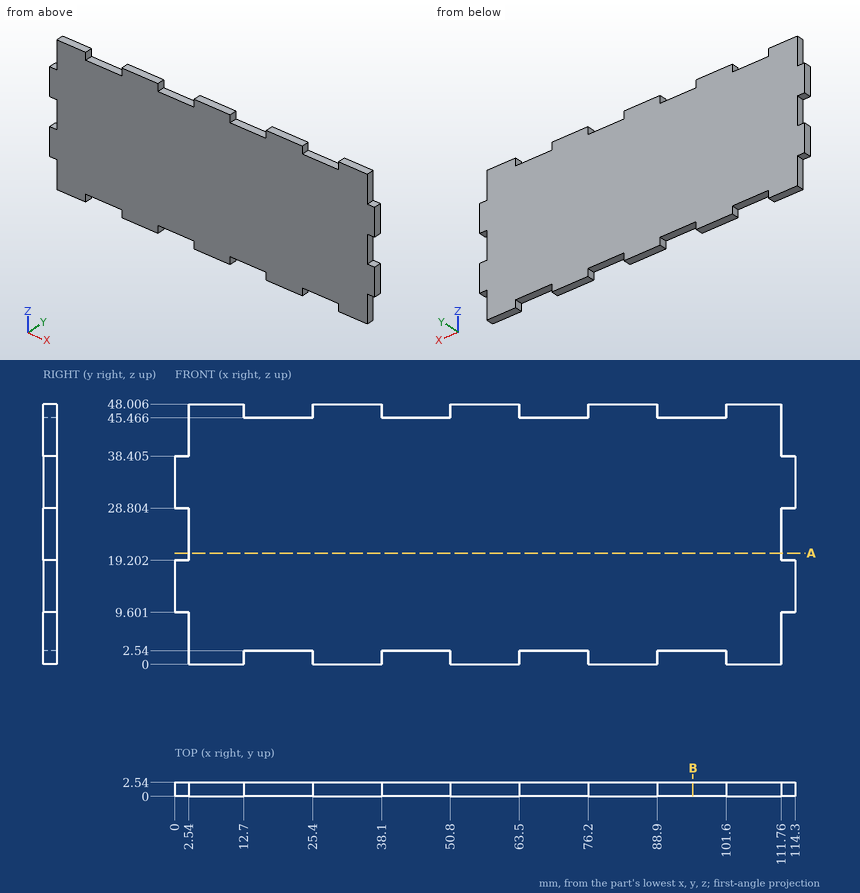
Design review of the part shown in the three views and the two pictorial views. Dimensions are in mm from the part's minimum x, y and z. Coordinates: 2 decimals unless noted, no trailing zeros. Write each loop counter-clockwise with the first axis right and the second up, starting at its lowest first coordinate (ties: lowest second). Pieces come first, ordered by that corner, then holes.
1) We need section A-A on z = 20.5. State the section outline as (x, y) points.
2) Clearance check with flat-ended pins moving along their axes: pin 1 Ø1.5 at (y, z) = (1, 21) entering from +X; pin 2 Ø0.8 at (x, y) = (43.5, 1.5) entering from +Z; pin 3 Ø0.8 at (x, y) = (113, 1.5) entering from -Z. State where each tip first meets the part, or that it passes through.
3) To check wall thickness, follow probe 1 along X at (y, z) = (1.55, 46.5); probe 2 along X at (y, z) = (1.65, 38.5); probe 3 along Z at (x, y) = (23, 2.3). State the ranges of each line that lie inside material, in increasing order.
4) We need section B-B on x = 95.5. State the section outline as (y, z) points, then the cut area to 3 significant figures.
Answer list:
1. outline: (2.54, 0) - (111.76, 0) - (111.76, 2.54) - (2.54, 2.54) - close
2. pin 1: stops at x = 111.76
2. pin 2: stops at z = 45.47
2. pin 3: stops at z = 9.6
3. probe 1: x = 2.54 to 12.7, 25.4 to 38.1, 50.8 to 63.5, 76.2 to 88.9, 101.6 to 111.76
3. probe 2: x = 2.54 to 111.76
3. probe 3: z = 2.54 to 45.47
4. outline: (0, 2.54) - (2.54, 2.54) - (2.54, 45.47) - (0, 45.47) - close
4. area: 109 mm2
